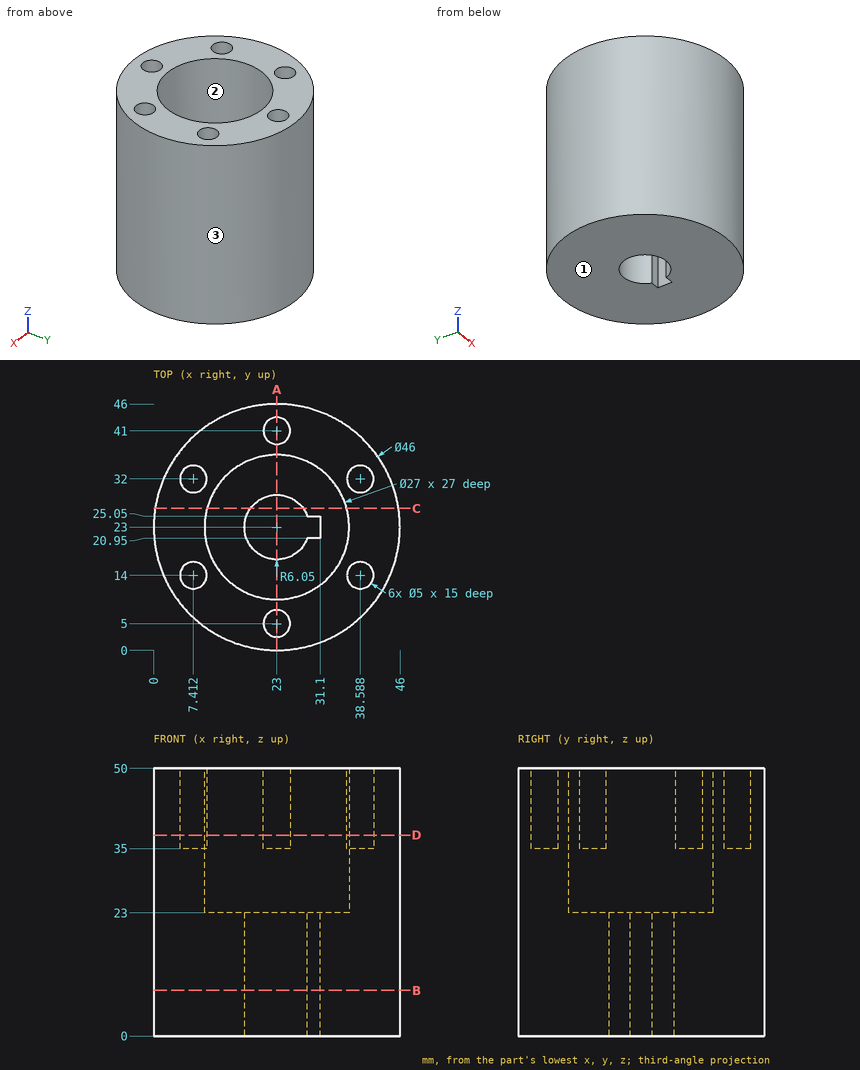
Can you work these out from the drawing? Everything is in mm from the part's minimum corner. Round coordinates to 2 decimals unless told otherwise and drop trailing zeros. Write each loop counter-clockwise with the first axis right and the second up, starting at its lowest first coordinate (ties: lowest second). Pieces come first, ordered by that corner, then holes.
1. Suppose I cut it at C-C (y = 26.5). List the corners of the cut face in (x, z) for me (1 decimal), and give its area (3 significant figures).
2. Will these pins go through, and if not, where does the flat tip stop? pin 1 Ø5 at (x, y) = (21.5, 25) entering from -Z; pin 2 Ø21.5 at (x, y) = (23, 23) entering from +Z; pin 3 Ø5 at (x, z) = (14, 31) entering from +Y; pin 4 Ø5 at (y, z) = (13, 23.5) entering from -X.
3. If we mould it in two halves opening along Y, with no side actions, what happens to the marked faces 1, 2 and 3? For each: released by +Y, released by -Y, zero draft, split by the parting line, or undercut.
4. I need wall thicknesses on L1, parallel to Y at x = 6, z = 40.5 (1 decimal); L2, parallel to X at y = 23.5, z = 31 (1 decimal); L3, parallel to Z at x = 37, y = 31.5. Which ranges of each line are inside material? Lowest first, please.
5. Suppose I cut it at A-A (x = 23). List the corners of the cut face in (y, z) for me.
6. Suppose I cut it at D-D (z = 37.5). List the corners of the cut face in (x, y) for me.
7. Suppose I cut it at B-B (z = 8.5). List the corners of the cut face in (x, y) for me, and give its area (3 significant figures).
Answer sheet:
1. outline: (0.3, 0) - (18.1, 0) - (18.1, 23) - (10, 23) - (10, 50) - (0.3, 50) - close; (27.9, 0) - (45.7, 0) - (45.7, 50) - (36, 50) - (36, 23) - (27.9, 23) - close
1. area: 1,340 mm2
2. pin 1: passes through
2. pin 2: stops at z = 23
2. pin 3: stops at y = 45.06
2. pin 4: stops at x = 1.26
3. face 1: zero draft
3. face 2: undercut
3. face 3: split by the parting line
4. L1: y = 7.5 to 11.9, 16.1 to 29.9, 34.1 to 38.5
4. L2: x = 0 to 9.5, 36.5 to 46
4. L3: z = 0 to 35
5. outline: (0, 0) - (16.95, 0) - (16.95, 23) - (9.5, 23) - (9.5, 50) - (7.5, 50) - (7.5, 35) - (2.5, 35) - (2.5, 50) - (0, 50) - close; (29.05, 0) - (46, 0) - (46, 50) - (43.5, 50) - (43.5, 35) - (38.5, 35) - (38.5, 50) - (36.5, 50) - (36.5, 23) - (29.05, 23) - close
6. outline: circle Ø46 at (23, 23); hole circle Ø5 at (7.41, 14); hole circle Ø5 at (7.41, 32); hole circle Ø27 at (23, 23); hole circle Ø5 at (23, 5); hole circle Ø5 at (23, 41); hole circle Ø5 at (38.59, 14); hole circle Ø5 at (38.59, 32)
7. outline: circle Ø46 at (23, 23); hole (17.31, 20.95) arc R6.05 ccw to (28.69, 20.95) - (31.1, 20.95) - (31.1, 25.05) - (28.69, 25.05) arc R6.05 ccw to (17.31, 25.05) arc R6.05 ccw to start
7. area: 1,540 mm2
